Design review of the part shown in the three views and the two pictorial views. Dimensions are in mm from the part's minimum x, y and z. A direction names the side the tool comes from. Give positions to 0.01 mm unless a question says otherwise; leave off trailing zeros. Loops run counter-clockwise (first coordinate to the right, second up) from the corner with the lowest first, then second, coordinate; pieces in that order, holes last.
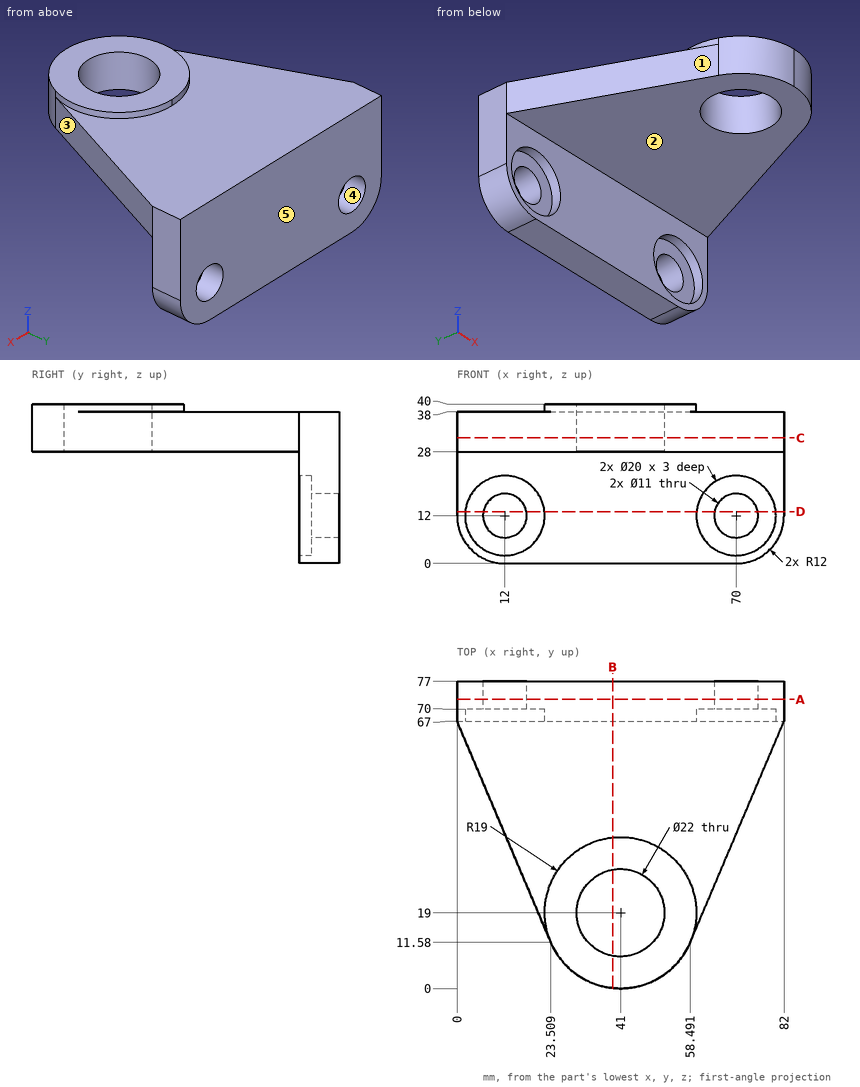
Q1. Consider section D-D on z = 13. Give the boundary of the cut face in (x, y).
Answers:
outline: (0, 67) - (2.05, 67) - (2.05, 70) - (6.59, 70) - (6.59, 77) - (0, 77) - close; (17.41, 70) - (21.95, 70) - (21.95, 67) - (60.05, 67) - (60.05, 70) - (64.59, 70) - (64.59, 77) - (17.41, 77) - close; (75.41, 70) - (79.95, 70) - (79.95, 67) - (82, 67) - (82, 77) - (75.41, 77) - close
Q2. Consider section A-A on y = 72.5. Give the boundary of the cut face in (x, z).
Answers:
outline: (0, 12) arc R12 ccw to (12, 0) - (70, 0) arc R12 ccw to (82, 12) - (82, 38) - (0, 38) - close; hole circle Ø11 at (12, 12); hole circle Ø11 at (70, 12)
Q3. Consider section C-C on z = 31.5. Give the boundary of the cut face in (x, y), plus the area to 3 significant figures.
Answers:
outline: (0, 67) - (23.51, 11.58) arc R19 ccw to (58.49, 11.58) - (82, 67) - (82, 77) - (0, 77) - close; hole circle Ø22 at (41, 19)
area: 3,970 mm2
Q4. For probe 1 along Z at (x, y) = (12, 69); probe 2 along Z at (x, y) = (12, 73); probe 3 along Y at (x, z) = (41, 33.5), list the stretches that pass through material, from the lowest coordinate up.
Answers:
probe 1: z = 0 to 2, 22 to 38
probe 2: z = 0 to 6.5, 17.5 to 38
probe 3: y = 0 to 8, 30 to 77
Q5. For pin 1 Ø4 at (x, z) = (35.5, 28) entering from -Y (1 decimal); pin 2 Ø1 at (x, z) = (52, 7) entering from -Y; pin 3 Ø20 at (x, y) = (53, 29) entering from -Z, all flat-tipped, find the tip position at first contact; note any pin that passes through.
Answers:
pin 1: stops at y = 0.3
pin 2: stops at y = 67
pin 3: stops at z = 28
Q6. Machinability: for the marked faces 1 and 2, which of the approach directions +Z, -Z, +X, -X, +Y, -Y give a long, thin tool a straight path to every point of the face, cutting with its end or side? Answer none if there is none.
Answers:
face 1: +Z, -Z, -X, -Y
face 2: -Z, +X, -X, -Y
Q7. Mouldability with a two-part tool opening along X and no side actions: class the marked faces 3, 4 and 5 as +X half, -X half, draft (parallel to the pull), parting line (faces both ways), or undercut.
Answers:
face 3: +X half
face 4: undercut
face 5: draft
Q8. Consider section B-B on x = 39. Give the boundary of the cut face in (y, z) (1 decimal), plus the area to 3 significant figures.
Answers:
outline: (0.1, 28) - (8.2, 28) - (8.2, 40) - (0.1, 40) - close; (29.8, 28) - (67, 28) - (67, 0) - (77, 0) - (77, 38) - (37.9, 38) - (37.9, 40) - (29.8, 40) - close
area: 865 mm2
